from build123d import *

# Parameters (mm, degrees)
SKETCH1_R                                           = 9.525
BOSS_EXTRUDE1_DEPTH                                 = 31.75
F_17_32_0_53125_DIAMETER_HOLE3_D                    = 16.03375
F_17_32_0_53125_DIAMETER_HOLE3_DEPTH                = 25.4
F_17_32_0_53125_DIAMETER_HOLE3_TIP                  = 4.817024475
CSK_FOR_1_4_FLAT_HEAD_MACHINE_SCREW_100_D           = 6.7564
CSK_FOR_1_4_FLAT_HEAD_MACHINE_SCREW_100_DEPTH       = 25.4
CSK_FOR_1_4_FLAT_HEAD_MACHINE_SCREW_100_CSINK_D     = 12.8778
CSK_FOR_1_4_FLAT_HEAD_MACHINE_SCREW_100_CSINK_ANGLE = 100
CSK_FOR_1_4_FLAT_HEAD_MACHINE_SCREW_100_TIP         = 2.029827343


with BuildPart() as part:
    # Sketch1 → Boss-Extrude1 (new body)
    with BuildSketch(Plane.XY):
        Circle(SKETCH1_R)
    extrude(amount=BOSS_EXTRUDE1_DEPTH)

    # 17/32 (0.53125) Diameter Hole3
    with Locations(Plane.XY.offset(31.75)):
        with Locations((0, 0)):
            Hole(F_17_32_0_53125_DIAMETER_HOLE3_D / 2, depth=F_17_32_0_53125_DIAMETER_HOLE3_DEPTH)
            with Locations((0, 0, -(F_17_32_0_53125_DIAMETER_HOLE3_DEPTH + F_17_32_0_53125_DIAMETER_HOLE3_TIP / 2))):  # 118° drill point
                Cone(0, F_17_32_0_53125_DIAMETER_HOLE3_D / 2, F_17_32_0_53125_DIAMETER_HOLE3_TIP, mode=Mode.SUBTRACT)

    # CSK for 1/4 Flat Head Machine Screw (100)1
    with Locations(Plane(origin=(0, 0, 0), x_dir=(-1, 0, 0), z_dir=(0, 0, -1))):
        with Locations((0, 0)):
            CounterSinkHole(CSK_FOR_1_4_FLAT_HEAD_MACHINE_SCREW_100_D / 2, CSK_FOR_1_4_FLAT_HEAD_MACHINE_SCREW_100_CSINK_D / 2, depth=CSK_FOR_1_4_FLAT_HEAD_MACHINE_SCREW_100_DEPTH, counter_sink_angle=CSK_FOR_1_4_FLAT_HEAD_MACHINE_SCREW_100_CSINK_ANGLE)
            with Locations((0, 0, -(CSK_FOR_1_4_FLAT_HEAD_MACHINE_SCREW_100_DEPTH + CSK_FOR_1_4_FLAT_HEAD_MACHINE_SCREW_100_TIP / 2))):  # 118° drill point
                Cone(0, CSK_FOR_1_4_FLAT_HEAD_MACHINE_SCREW_100_D / 2, CSK_FOR_1_4_FLAT_HEAD_MACHINE_SCREW_100_TIP, mode=Mode.SUBTRACT)


solid = part.part
The model under review builds one solid part; all positions refer to its coordinate system, in mm. A direction names the side the tool comes from. Give positions to 0.01 mm unless a question says otherwise; leave off trailing zeros. Loops run counter-clockwise (first coordinate to the right, second up) from the corner with the lowest first, then second, coordinate; pieces in that order, holes last. Notation, with made-up numbers: (43.5, 13.25) -> (81.5, 13.25) arc R32 cw to (81.5, 44.25) -> close; hole circle Ø2 at (35.5, 4). An arc over 180 degrees is marked (long way). Answer as a JSON object with one key per item and string values. Group by question number.
Q1. Take a section at C-C (z = 17). Write out the cut boundary in (x, y) (3 decimals), plus the area to 3 significant figures.
Q2. Wall thickness on line 1 along Y through (x, z) = (0, 2.95) (3 decimals); line 2 along Y through (x, z) = (-2.75, 9); line 3 along X through (y, z) = (1.5, 3.5): over which ranges is each line inside the solid? List them lowest first.
Q3. Take a section at A-A (x = 0). Write out the cut boundary in (y, z) (3 decimals).
Q4. Insertion check: pin 1 (2 mm diameter, centred on x = 5, y = 0, fed in from -Z); pin 2 (3 mm diameter, centred on x = 5.5, z = 18.5, fed in from +Y); pin 3 (8 mm diameter, centred on x = 0, y = 0, fed in from -Z). Each pin has a flat end and moves straight along its axis. Give the tip position at first contact, or say it passes through.
Q5. Tool access review of faces 1 (the cylindrical face through (-7.647, 2.408, 18.872)), 2 (the flat face through (-4.3, -7, 31.75)): name each direction out of +Z, -Z, +X, -X, +Y, -Y from which nothing blocks a thin tool from reaching the whole face with its end or side.
Answer below:
{
 "1": {"outline": "circle Ø19.05 at (0, 0); hole circle Ø16.034 at (0, 0)", "area": "83.1 mm2"},
 "2": {"line 1": "y = -9.525 to -3.378, 3.378 to 9.525", "line 2": "y = -9.12 to -7.53, 7.53 to 9.12", "line 3": "x = -9.41 to -3.03, 3.03 to 9.41"},
 "3": {"outline": "(-9.525, 0) -> (-6.439, 0) -> (-3.378, 2.568) -> (-3.378, 3.563) -> (-8.017, 6.35) -> (-8.017, 31.75) -> (-9.525, 31.75) -> close; (3.378, 2.568) -> (6.439, 0) -> (9.525, 0) -> (9.525, 31.75) -> (8.017, 31.75) -> (8.017, 6.35) -> (3.378, 3.563) -> close"},
 "4": {"pin 1": "stops at z = 0.37", "pin 2": "stops at y = 8.64", "pin 3": "stops at z = 2.05"},
 "5": {"face 1": "+Z", "face 2": "+Z, +X, -X, +Y, -Y"}
}
